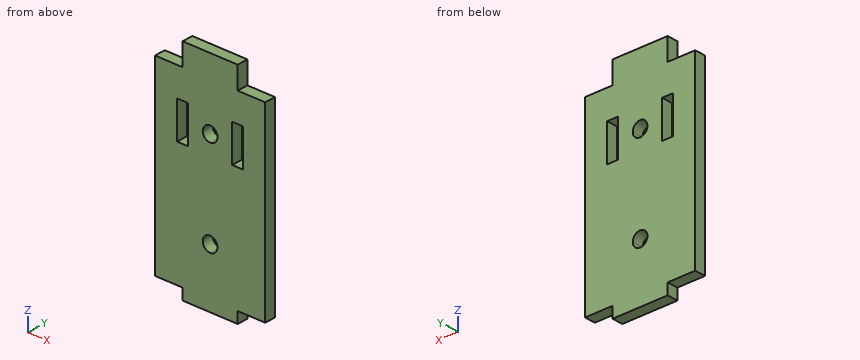
```python
from build123d import *

# Parameters (mm, degrees)
SKETCH1_W           = 7.5
SKETCH1_H           = 6
BOSS_EXTRUDE1_DEPTH = 3


with BuildPart() as part:
    # Sketch1 → Boss-Extrude1 (new body)
    with BuildSketch(Plane(origin=(0, 0, 0), x_dir=(1, 0, 0), z_dir=(0, 1, 0))):
        with BuildLine():
            Line((0, 14.75), (0, 25.5))
            Line((0, 25.5), (-7.5, 25.5))
            Line((-7.5, 25.5), (-15, 25.5))
            Line((-15, 25.5), (-15, -12.75))
            Line((-15, -12.75), (-9, -12.75))
            Line((-9, -12.75), (-9, -7.75))
            Line((-9, -7.75), (-6, -7.75))
            Line((-6, -7.75), (-6, -12.75))
            Line((-6, -12.75), (-2, -12.75))
            ThreePointArc((-2, -12.75), (-1.414213562, -11.335786438), (0, -10.75))
            Line((0, -10.75), (0, 0))
            Line((0, 0), (0, 10.75))
            ThreePointArc((0, 10.75), (-2, 12.75), (0, 14.75))
        make_face()
        with BuildLine():
            Line((-9, -12.75), (-15, -12.75))
            Line((-15, -12.75), (-15, -25.5))
            Line((-15, -25.5), (-7.5, -25.5))
            Line((-7.5, -25.5), (0, -25.5))
            Line((0, -25.5), (0, -14.75))
            ThreePointArc((0, -14.75), (-1.414213562, -14.164213562), (-2, -12.75))
            Line((-2, -12.75), (-6, -12.75))
            Line((-6, -12.75), (-6, -17.75))
            Line((-6, -17.75), (-9, -17.75))
            Line((-9, -17.75), (-9, -12.75))
        make_face()
        with BuildLine():
            Line((15, -25.5), (15, -12.75))
            Line((15, -12.75), (9, -12.75))
            Line((9, -12.75), (9, -17.75))
            Line((9, -17.75), (6, -17.75))
            Line((6, -17.75), (6, -12.75))
            Line((6, -12.75), (2, -12.75))
            ThreePointArc((2, -12.75), (1.414213562, -14.164213562), (0, -14.75))
            Line((0, -14.75), (0, -25.5))
            Line((0, -25.5), (7.5, -25.5))
            Line((7.5, -25.5), (15, -25.5))
        make_face()
        with BuildLine():
            Line((7.5, 25.5), (0, 25.5))
            Line((0, 25.5), (0, 14.75))
            ThreePointArc((0, 14.75), (1.414213562, 14.164213562), (2, 12.75))
            ThreePointArc((2, 12.75), (1.414213562, 11.335786438), (0, 10.75))
            Line((0, 10.75), (0, 0))
            Line((0, 0), (0, -10.75))
            ThreePointArc((0, -10.75), (1.414213562, -11.335786438), (2, -12.75))
            Line((2, -12.75), (6, -12.75))
            Line((6, -12.75), (6, -7.75))
            Line((6, -7.75), (9, -7.75))
            Line((9, -7.75), (9, -12.75))
            Line((9, -12.75), (15, -12.75))
            Line((15, -12.75), (15, 25.5))
            Line((15, 25.5), (7.5, 25.5))
        make_face()
        Polygon((-7.5, 25.5), (0, 25.5), (7.5, 25.5), (7.5, 28.5), (-7.5, 28.5), align=None)
        Polygon((-7.5, 25.5), (0, 25.5), (7.5, 25.5), (7.5, 28.5), (-7.5, 28.5), align=None)
        with Locations((-3.75, -28.5)):
            Rectangle(SKETCH1_W, SKETCH1_H)
        with Locations((3.75, -28.5)):
            Rectangle(SKETCH1_W, SKETCH1_H)
    extrude(amount=BOSS_EXTRUDE1_DEPTH)


solid = part.part
```
Source: CAD feature listing. Evaluate the final solid. Frame: model axes, mm. Round coordinates to 2 decimals unless told otherwise and drop trailing zeros. Loops run counter-clockwise (first coordinate to the right, second up) from the corner with the lowest first, then second, coordinate; pieces in that order, holes last.
1. Section query C-C on z = 27. Output: boundary loops of the cut face in (x, y).
2. Section query D-D on x = -11. Output: boundary loops of the cut face in (y, z), and give its area (3 significant figures).
3. Ray query, L1, parallel to X at y = 2.7, z = 8.5; L2, parallel to Z at x = -6.5, y = 2.35; L3, parallel to Z at x = 0.25, y = 2.45. Return the intervals inside material, ascending.
4. Section query A-A on z = 9. Output: boundary loops of the cut face in (x, y), and give its area (3 significant figures).
5. Section query B-B on y = 1.35. Output: boundary loops of the cut face in (x, z).
6. Contact query for flat-ended pins moving along their axis: pin 1 (1.5 mm diameter, centred on x = -10, y = 1.5, fed in from -Z); pin 2 (0.9 mm diameter, centred on y = 1, z = -27, fed in from -X); pin 3 (0.9 mm diameter, centred on y = 1.5, z = -26.5, fed in from +X). Output: stop coordinate, or through.
Answers below:
1. outline: (-7.5, 0) - (7.5, 0) - (7.5, 3) - (-7.5, 3) - close
2. outline: (0, -25.5) - (3, -25.5) - (3, 25.5) - (0, 25.5) - close
2. area: 153 mm2
3. L1: x = -15 to -9, -6 to 6, 9 to 15
3. L2: z = -28.5 to 7.75, 17.75 to 31.5
3. L3: z = -28.5 to -14.73, -10.77 to 10.77, 14.73 to 31.5
4. outline: (-15, 0) - (-9, 0) - (-9, 3) - (-15, 3) - close; (-6, 0) - (6, 0) - (6, 3) - (-6, 3) - close; (9, 0) - (15, 0) - (15, 3) - (9, 3) - close
4. area: 72.0 mm2
5. outline: (-15, -25.5) - (-7.5, -25.5) - (-7.5, -28.5) - (7.5, -28.5) - (7.5, -25.5) - (15, -25.5) - (15, 25.5) - (7.5, 25.5) - (7.5, 31.5) - (-7.5, 31.5) - (-7.5, 25.5) - (-15, 25.5) - close; hole (-9, 7.75) - (-6, 7.75) - (-6, 17.75) - (-9, 17.75) - close; hole circle Ø4 at (0, -12.75); hole circle Ø4 at (0, 12.75); hole (6, 7.75) - (9, 7.75) - (9, 17.75) - (6, 17.75) - close
6. pin 1: stops at z = -25.5
6. pin 2: stops at x = -7.5
6. pin 3: stops at x = 7.5
